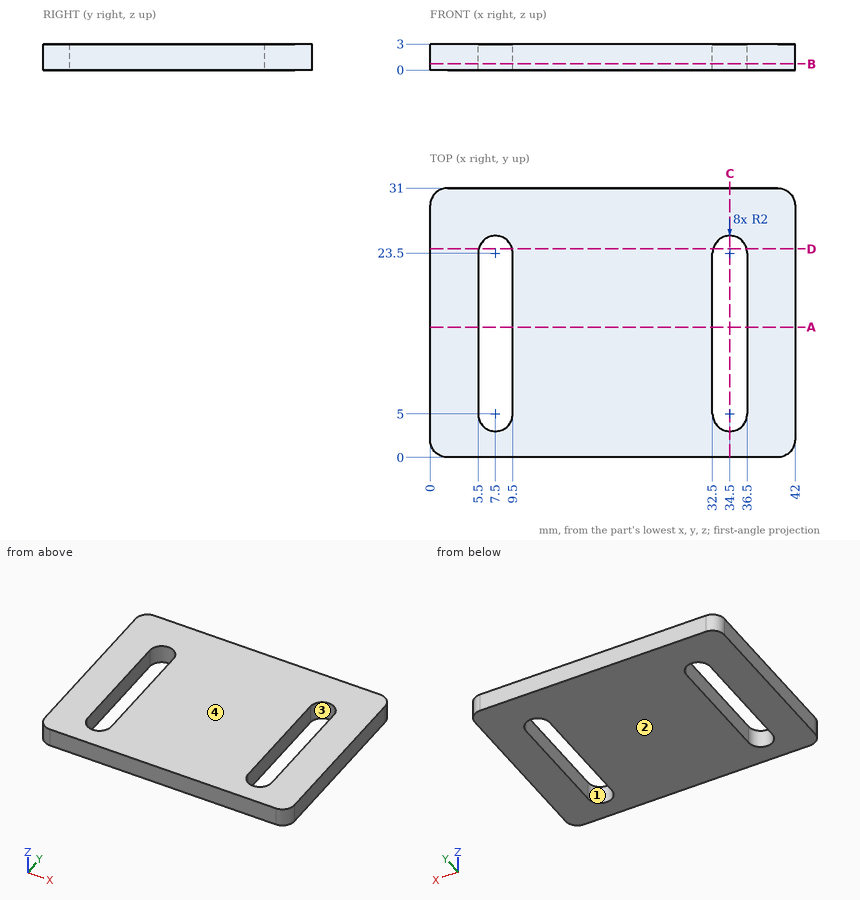
Study the drawing (mm; zero at the part's minimum x, y, z) and answer. A direction names the side the tool comes from. Coordinates: 2 decimals unless noted, no trailing zeros. Loops run counter-clockwise (first coordinate to the right, second up) from the corner with the lowest first, then second, coordinate; pieces in that order, holes last. Notation, with made-up numbers: M 62,-17.75 L 116,-17.75 A10 cw 116,-6.75 Z; hole C -10,75 d8. An arc over 180 degrees is marked long. Answer in a Markdown table with one row per item. Add a question column.
1. The mould has two halves that part along Y. Classify the marked faces 3 and 4: pulls with the +Y half, pulls with the -Y half, needs draft (parallel to the pull), parting line crosses it, or undercut.
2. Find section C-C, the plane x = 34.5. Write down the section's boundary in (y, z).
3. Find section D-D, the plane y = 24. Write down the section's boundary in (x, z).
4. Find section B-B, the plane z = 0.7. Write down the section's boundary in (x, y), then the cut area to 3 significant figures.
5. A tool of negligible diameter and unlimited length cuts with its end or side. For the marked faces 1 and 2, from which of +Z, -Z, +X, -X, +Y, -Y can it reach the whole face along a straight path? Write none if from no direction.
6. Consider L1, parallel to X at y = 8.5, z = 2.7; L2, parallel to X at y = 24.5, z = 2.45; L3, parallel to Y at x = 34, z = 2.15. Determine where each line is inside the solid, lowest interval first.
7. Find section A-A, the plane y = 15. Write down the section's boundary in (x, z).
Reported:
| question | item | result |
|---|---|---|
| 1 | face 3 | undercut |
| 1 | face 4 | needs draft |
| 2 | outline | M 0,0 L 3,0 L 3,3 L 0,3 Z; M 25.5,0 L 31,0 L 31,3 L 25.5,3 Z |
| 3 | outline | M 0,0 L 5.56,0 L 5.56,3 L 0,3 Z; M 9.44,0 L 32.56,0 L 32.56,3 L 9.44,3 Z; M 36.44,0 L 42,0 L 42,3 L 36.44,3 Z |
| 4 | outline | M 0,2 A2 ccw 2,0 L 40,0 A2 ccw 42,2 L 42,29 A2 ccw 40,31 L 2,31 A2 ccw 0,29 Z; hole M 5.5,5 A2 ccw 9.5,5 L 9.5,23.5 A2 ccw 5.5,23.5 Z; hole M 32.5,5 A2 ccw 36.5,5 L 36.5,23.5 A2 ccw 32.5,23.5 Z |
| 4 | area | 1,130 mm^2 |
| 5 | face 1 | +Z, -Z |
| 5 | face 2 | -Z, +X, -X, +Y, -Y |
| 6 | L1 | x = 0 to 5.5, 9.5 to 32.5, 36.5 to 42 |
| 6 | L2 | x = 0 to 5.77, 9.23 to 32.77, 36.23 to 42 |
| 6 | L3 | y = 0 to 3.06, 25.44 to 31 |
| 7 | outline | M 0,0 L 5.5,0 L 5.5,3 L 0,3 Z; M 9.5,0 L 32.5,0 L 32.5,3 L 9.5,3 Z; M 36.5,0 L 42,0 L 42,3 L 36.5,3 Z |
